Design review of the part shown in the three views and the two pictorial views. Dimensions are in mm from the part's minimum x, y and z. Give positions to 0.01 mm unless a question says otherwise; leave off trailing zeros. Write each loop counter-clockwise with the first axis right and the second up, starting at its lowest first coordinate (ties: lowest second). Pieces come first, ordered by that corner, then holes. Notation, with made-up numbers: (28, -17) -> (81, -17) arc R29 ccw to (81, 11) -> close; hole circle Ø2 at (4, 14.25). An arc over 180 degrees is marked (long way). Use CSV: the item, a comma, the result in double quotes.
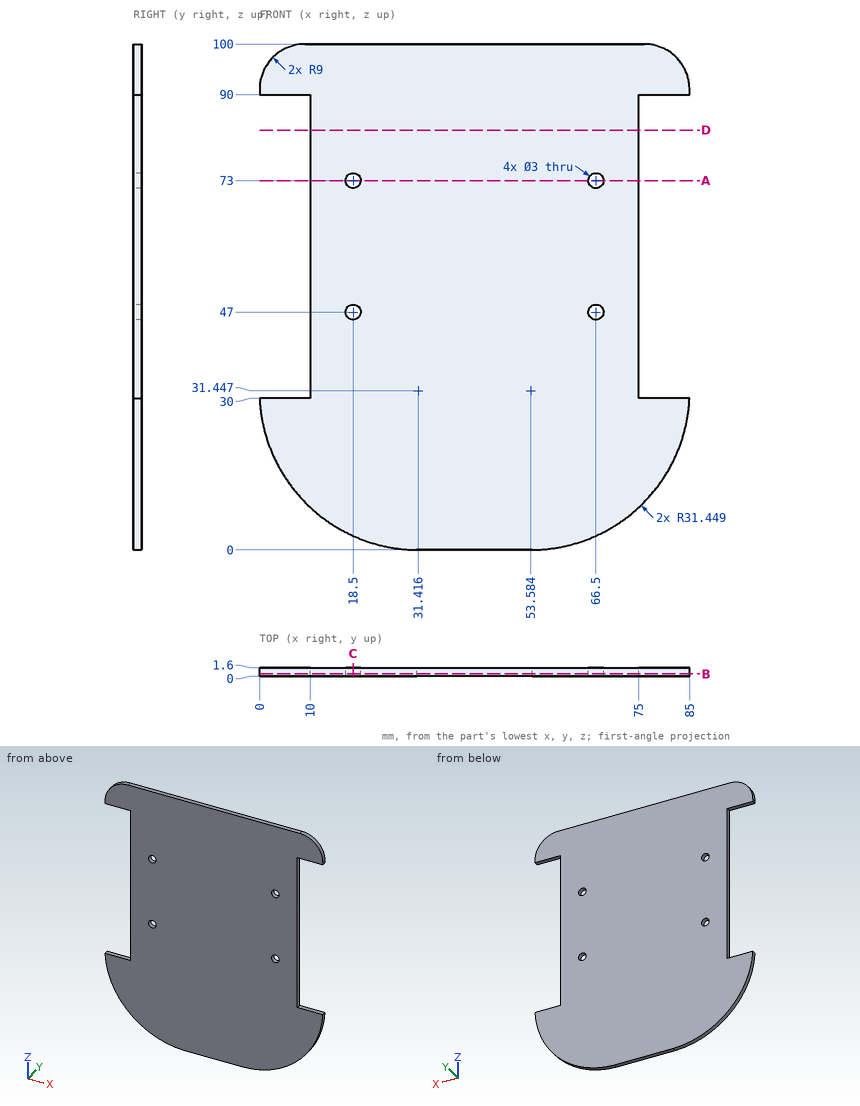
Q1. Insertion check: pin 1 (0.5 mm diameter, centred on x = 79.5, y = 0.5, fed in from -Z); pin 2 (0.8 mm diameter, centred on x = 7, y = 1, fed in from +Z); pin 3 (0.5 mm diameter, centred on y = 0.5, z = 73.5, fed in from +X); pin 4 (1.8 mm diameter, centred on x = 18.5, z = 47, fed in from -Y). Each pin has a flat end and moves straight along its axis. Give the tip position at first contact, or say it passes through.
Derived:
pin 1,"stops at z = 13.27"
pin 2,"stops at z = 99.86"
pin 3,"stops at x = 75"
pin 4,"passes through"
Q2. Consider section C-C (x = 18.5). Write out the cut boundary in (y, z).
Derived:
outline,"(0, 2.77) -> (1.6, 2.77) -> (1.6, 45.5) -> (0, 45.5) -> close; (0, 48.5) -> (1.6, 48.5) -> (1.6, 71.5) -> (0, 71.5) -> close; (0, 74.5) -> (1.6, 74.5) -> (1.6, 100) -> (0, 100) -> close"
Q3. Consider section B-B (y = 0.4). Write out the cut boundary in (x, z).
Derived:
outline,"(0, 30) arc R31.45 ccw to (31.06, 0) -> (53.94, 0) arc R31.45 ccw to (85, 30) -> (75, 30) -> (75, 90) -> (85, 90) -> (85, 91) arc R9 ccw to (76, 100) -> (9, 100) arc R9 ccw to (0, 91) -> (0, 90) -> (10, 90) -> (10, 30) -> close; hole circle Ø3 at (18.5, 47); hole circle Ø3 at (18.5, 73); hole circle Ø3 at (66.5, 47); hole circle Ø3 at (66.5, 73)"
Q4. To check wall thickness, follow probe 1 along X at (y, z) = (1, 47); probe 2 along Z at (x, y) = (66.5, 1.2); probe 3 along X at (y, z) = (0.85, 48). State the ranges of each line that lie inside material, in increasing order.
Derived:
probe 1,"x = 10 to 17, 20 to 65, 68 to 75"
probe 2,"z = 2.77 to 45.5, 48.5 to 71.5, 74.5 to 100"
probe 3,"x = 10 to 17.38, 19.62 to 65.38, 67.62 to 75"
Q5. Consider section A-A (z = 73). Write out the cut boundary in (x, y), then the cut area to 3 significant figures.
Derived:
outline,"(10, 0) -> (17, 0) -> (17, 1.6) -> (10, 1.6) -> close; (20, 0) -> (65, 0) -> (65, 1.6) -> (20, 1.6) -> close; (68, 0) -> (75, 0) -> (75, 1.6) -> (68, 1.6) -> close"
area,"94.4 mm2"
Q6. Consider section D-D (z = 83). Write out the cut boundary in (x, y), then the cut area to 3 significant figures.
Derived:
outline,"(10, 0) -> (75, 0) -> (75, 1.6) -> (10, 1.6) -> close"
area,"104 mm2"
